Design review of the part built by this model. Coordinates are the model's own, in mm. A direction names the side the tool comes from. Coordinates: 2 decimals unless noted, no trailing zeros. Order: outer loops, then holes, each group sorted by start corner. A loop starts at its lowest first (then second) coordinate and runs counter-clockwise, first axis right, second up.
from build123d import *

# Parameters (mm, degrees)
SKETCH1_W               = 15.7
SKETCH1_H               = 28.6
BODY_DEPTH              = 24.3
SKETCH2_R               = 5.953125
PANEL_MOUNT_15_32_DEPTH = 12.2
SWITCH_DEPTH            = 3.048
SWITCH_DEPTH_BACK       = 2.54
SKETCH10_W              = 0.8
SKETCH10_H              = 6.3
CONNECTORS_DEPTH        = 10.8


with BuildPart() as part:
    # Sketch1 → Body (new body)
    with BuildSketch(Plane(origin=(0, 0, 0), x_dir=(1, 0, 0), z_dir=(0, 1, 0))):
        Rectangle(SKETCH1_W, SKETCH1_H)
    extrude(amount=BODY_DEPTH)

    # Sketch2 → Panel Mount  15/32 (add)
    with BuildSketch(Plane(origin=(0, 24.3, 0), x_dir=(1, 0, 0), z_dir=(0, 1, 0))):
        Circle(SKETCH2_R)
    extrude(amount=PANEL_MOUNT_15_32_DEPTH)

    # Sketch9 → Switch (add, two sides)
    with BuildSketch(Plane(origin=(0, 0, 0), x_dir=(0, 0, -1), z_dir=(1, 0, 0))) as switch_sk:
        with BuildLine():
            Line((0, 36.5), (-6, 36.5))
            Line((-6, 36.5), (-9.40084725, 52.842068887))
            ThreePointArc((-9.40084725, 52.842068887), (-6.42619484, 55.699919466), (-3.409982549, 52.885966675))
            Line((-3.409982549, 52.885966675), (0, 36.5))
        make_face()
    extrude(amount=SWITCH_DEPTH)
    extrude(switch_sk.sketch, amount=-SWITCH_DEPTH_BACK)

    # Sketch10 → Connectors (add)
    with BuildSketch(Plane.XZ):
        Polygon((-6.390931504, 8.976782117), (-5.891175466, 8.352087069), (-0.971701967, 12.287665869), (-1.471458005, 12.912360916), align=None)
        Rectangle(SKETCH10_W, SKETCH10_H)
    extrude(amount=CONNECTORS_DEPTH)


solid = part.part
1. Add section C-C (x = -3.5). Give the boundary of the cut face in (y, z), and give its area (3 significant figures).
2. Insertion check: pin 1 (1 mm diameter, centred on x = -1, z = 5.5, fed in from -Y); pin 2 (1.9 mm diameter, centred on y = -6.5, z = 1, fed in from -X); pin 3 (8 mm diameter, centred on y = 45.5, z = 8.5, fed in from -X); pin 4 (8 mm diameter, centred on x = 1.5, z = 0, fed in from -Y). Each pin has a flat end and moves straight along its axis. Give the tip position at first contact, or say it passes through.
3. Add section A-A (y = -2.5). Give the boundary of the cut face in (x, z), and give its area (3 significant figures).
4. For faces 1 (the flat face through (-3.9, -5.32, 10.97)), 2 (the flat face through (-2.54, 46, 5)), 3 (the flat face through (0.4, -5, 0)), 4 (the flat face through (0.293, 44.557, 7.677)), list the 3-axis set-ups (+Z, -Z, +X, -X, +Y, -Y) from which the entire face can be reached by the end or side of a thin tool; tool diameter is ignored.
5. Mouldability with a two-part tool opening along Y and no side actions: class faces 5 (the cylindrical face through (-4.724, 30.315, 3.622)), 6 (the flat face through (0.29, 44.81, 1.73)), 7 (the flat face through (0, 12, -14.3)) as pulls with the +Y half, pulls with the -Y half, needs draft (parallel to the pull), parting line crosses it, or undercut.
6. To check wall thickness, follow line 1 (Y direction, x = 2.5, z = -5.25); line 2 (Y direction, x = 0.5, z = 10.5); line 3 (Z direction, x = 0, y = 50). State the ranges of each line that lie inside material, in increasing order.
7. Add section B-B (z = 2). Give the boundary of the cut face in (x, y).
8. Add section D-D (y = 26). Give the boundary of the cut face in (x, z).
Solution:
1. outline: (-10.8, 10.27) - (0, 10.27) - (0, -14.3) - (24.3, -14.3) - (24.3, -4.82) - (36.5, -4.82) - (36.5, 4.82) - (24.3, 4.82) - (24.3, 14.3) - (0, 14.3) - (0, 11.29) - (-10.8, 11.29) - close
1. area: 824 mm2
2. pin 1: stops at y = 0
2. pin 2: stops at x = -0.4
2. pin 3: stops at x = -2.54
2. pin 4: stops at y = -10.8
3. outline: (-6.39, 8.98) - (-5.89, 8.35) - (-0.97, 12.29) - (-1.47, 12.91) - close; (-0.4, -3.15) - (0.4, -3.15) - (0.4, 3.15) - (-0.4, 3.15) - close
3. area: 10.1 mm2
4. face 1: +Z, -X, -Y
4. face 2: +Z, -Z, -X, +Y
4. face 3: +Z, -Z, +X, -Y
4. face 4: +Z, +X, -X
5. face 5: undercut
5. face 6: pulls with the +Y half
5. face 7: needs draft
6. line 1: y = 0 to 36.5
6. line 2: y = 0 to 24.3
6. line 3: z = 2.81 to 8.81
7. outline: (-7.85, 0) - (-0.4, 0) - (-0.4, -10.8) - (0.4, -10.8) - (0.4, 0) - (7.85, 0) - (7.85, 24.3) - (5.61, 24.3) - (5.61, 36.5) - (3.05, 36.5) - (3.05, 46.11) - (-2.54, 46.11) - (-2.54, 36.5) - (-5.61, 36.5) - (-5.61, 24.3) - (-7.85, 24.3) - close
8. outline: circle Ø11.91 at (0, 0)
